Source: CAD feature listing. Evaluate the final solid. Frame: model axes, mm. Face numbers are marked on the shaded views. A direction names the side the tool comes from. Round coordinates to 2 decimals unless told otherwise and drop trailing zeros. Write each loop counter-clockwise with the first axis right and the second up, starting at its lowest first coordinate (ties: lowest second). Pieces come first, ordered by that corner, then holes.
```python
from build123d import *

# Parameters (mm, degrees)
EXTRU_MINCE1_DEPTH      = 53
ENL_V_MAT_EXTRU_1_DEPTH = 57.384838388
ESQUISSE3_R             = 1.1
ENL_V_MAT_EXTRU_2_DEPTH = 55.351611691


with BuildPart() as part:
    # Esquisse1 → Extru.-Mince1 (new body)
    with BuildSketch(Plane.XY):
        with BuildLine():
            Line((-9.5, 0), (-2.5, 0))
            Line((-2.5, 0), (-2.5, 4.5))
            ThreePointArc((-2.5, 4.5), (0, 7), (2.5, 4.5))
            Line((2.5, 4.5), (2.5, 0))
            Line((2.5, 0), (17.5, 0))
            Line((17.5, 0), (17.5, 1))
            Line((17.5, 1), (3.5, 1))
            Line((3.5, 1), (3.5, 4.5))
            ThreePointArc((3.5, 4.5), (0, 8), (-3.5, 4.5))
            Line((-3.5, 4.5), (-3.5, 1))
            Line((-3.5, 1), (-9.5, 1))
            Line((-9.5, 1), (-9.5, 0))
        make_face()
    extrude(amount=EXTRU_MINCE1_DEPTH)

    # Esquisse2 → Enlèv. mat.-Extru.1 (cut, through all)
    with BuildSketch(Plane(origin=(0, 0, 0), x_dir=(1, 0, 0), z_dir=(0, 1, 0))):
        Polygon((2.5, 0), (-9.5, -8.402490459), (-9.5, 0), align=None)
        Polygon((17.5, -53), (17.5, 61.57469904), (3.177754145, -53), align=None)
        Polygon((-9.5, -48.798754771), (-9.5, -53), (-3.5, -53), align=None)
    extrude(amount=ENL_V_MAT_EXTRU_1_DEPTH, mode=Mode.SUBTRACT)

    # Esquisse3 → Enlèv. mat.-Extru.2 (cut, through all)
    with BuildSketch(Plane(origin=(0, 1, 0), x_dir=(1, 0, 0), z_dir=(0, 1, 0))):
        with Locations(Location((-7, -28.600622615, 0), (0, 0, 270))):
            Circle(ESQUISSE3_R)
    extrude(amount=-ENL_V_MAT_EXTRU_2_DEPTH, mode=Mode.SUBTRACT)


solid = part.part
```
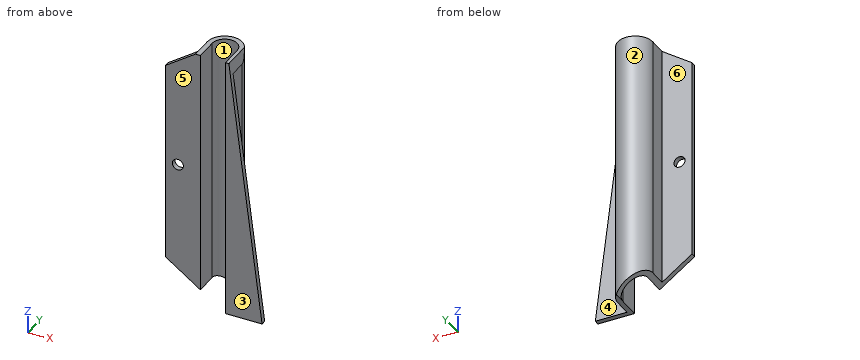
Q1. Pin query (flat end, axial travel): P1, Ø2, axis at y = 3.5, z = 45.5, coming from the -X side; P2, Ø3, axis at x = 6, y = 5.5, coming from the +Z side; P3, Ø1.9, axis at x = 5.5, z = 20, coming from the +Y side; P4, Ø1, axis at x = -1, z = 18, coming from the -Y side. Return the tip coordinate at first contact, or that it passes through.
Q2. Set-up query: the marked faces 4, 5 and 6. Return all of +Z, -Z, +X, -X, +Y, -Y with unobstructed straight access to the full face (end or side cutting, diameter ignored); none if empty.
Q3. Section query A-A, the plane y = 3.75. Output: boundary loops of the cut face in (x, z).
Q4. Section query D-D, the plane z = 9. Output: boundary loops of the cut face in (x, y).
Q5. Section query C-C, the plane z = 26. Output: boundary loops of the cut face in (x, y), and give its area (3 significant figures).
Q6. Line query: line 1 (X direction, y = 2.5, z = 43); line 2 (Y direction, x = -4.5, z = 12); line 3 (X direction, y = 0.5, z = 13.5). Output: solid intervals per line, ascending.
Q7. Mould query, pull axis X, two halves, no side actions, for the marked faces 1, 2 and 3. Classes: pulls with the +X half, pulls with the -X half, needs draft (parallel to the pull), parting line crosses it, or undercut.
Q8. Section query B-B, the plane x = -7. Output: boundary loops of the cut face in (y, z), and give its area (3 significant figures).
Filled in:
1. P1: stops at x = -3.5
1. P2: passes through
1. P3: stops at y = 1
1. P4: stops at y = 6.5
2. face 4: +Z, -Z, +X, +Y
2. face 5: +Z, -Z, +X, -X, -Y
2. face 6: +Z, -Z, -X, +Y
3. outline: (-3.5, 4.2) - (-2.5, 3.5) - (-2.5, 53) - (-3.5, 53) - close; (2.5, 0) - (3.5, 0) - (3.5, 50.42) - (3.18, 53) - (2.5, 53) - close
4. outline: (-9.5, 0) - (-2.5, 0) - (-2.5, 4.5) arc R2.5 cw to (2.5, 4.5) - (2.5, 0) - (8.68, 0) - (8.68, 1) - (3.5, 1) - (3.5, 4.5) arc R3.5 ccw to (-3.5, 4.5) - (-3.5, 1) - (-9.5, 1) - close
5. outline: (-9.5, 0) - (-2.5, 0) - (-2.5, 4.5) arc R2.5 cw to (2.5, 4.5) - (2.5, 0) - (6.55, 0) - (6.55, 1) - (3.5, 1) - (3.5, 4.5) arc R3.5 ccw to (-3.5, 4.5) - (-3.5, 1) - (-9.5, 1) - close
5. area: 27.5 mm2
6. line 1: x = -3.5 to -2.5, 2.5 to 3.5
6. line 2: y = 0 to 1
6. line 3: x = -9.5 to -2.5, 2.5 to 8.12
7. face 1: undercut
7. face 2: parting line crosses it
7. face 3: needs draft
8. outline: (0, 6.65) - (1, 6.65) - (1, 27.5) - (0, 27.5) - close; (0, 29.7) - (1, 29.7) - (1, 50.55) - (0, 50.55) - close
8. area: 41.7 mm2
